```python
from build123d import *

# Parameters (mm, degrees)
SKETCH2_W                                           = 70
SKETCH2_H                                           = 115
BOSS_EXTRUDE1_DEPTH                                 = 10
SKETCH8_W                                           = 70
SKETCH8_H                                           = 77
SKETCH8_W_2                                         = 44
SKETCH8_H_2                                         = 59
BOSS_EXTRUDE5_DEPTH                                 = 50
SKETCH9_R                                           = 4
CUT_EXTRUDE1_DEPTH                                  = 50
CUT_EXTRUDE2_REACH                                  = 107.948
SKETCH10_W                                          = 25
SKETCH10_H                                          = 25
CSK_FOR_M3_COUNTERSUNK_FLAT_HEAD_SCREW1_D           = 3.4
CSK_FOR_M3_COUNTERSUNK_FLAT_HEAD_SCREW1_DEPTH       = 5
CSK_FOR_M3_COUNTERSUNK_FLAT_HEAD_SCREW1_CSINK_D     = 6.3
CSK_FOR_M3_COUNTERSUNK_FLAT_HEAD_SCREW1_CSINK_ANGLE = 90
FILLET1_R                                           = 2
CSK_FOR_M3_COUNTERSUNK_FLAT_HEAD_SCR_2_COUNT        = 2
CSK_FOR_M3_COUNTERSUNK_FLAT_HEAD_SCR_2_PITCH        = 59.993922781
CSK_FOR_M3_COUNTERSUNK_FLAT_HEAD_SCR_3_COUNT        = 2
CSK_FOR_M3_COUNTERSUNK_FLAT_HEAD_SCR_3_PITCH        = 84.983361201
CSK_FOR_M3_COUNTERSUNK_FLAT_HEAD_SCR_4_COUNT        = 2
CSK_FOR_M3_COUNTERSUNK_FLAT_HEAD_SCR_4_PITCH        = 102.955177918
CSK_FOR_M3_COUNTERSUNK_FLAT_HEAD_SCR_5_COUNT        = 2
CSK_FOR_M3_COUNTERSUNK_FLAT_HEAD_SCR_5_PITCH        = 118.101251225
CSK_FOR_M3_COUNTERSUNK_FLAT_HEAD_SCR_6_COUNT        = 2
CSK_FOR_M3_COUNTERSUNK_FLAT_HEAD_SCR_6_PITCH        = 102.856688561
CSK_FOR_M5_COUNTERSUNK_FLAT_HEAD_SCREW2_D           = 5.5
CSK_FOR_M5_COUNTERSUNK_FLAT_HEAD_SCREW2_DEPTH       = 30
CSK_FOR_M5_COUNTERSUNK_FLAT_HEAD_SCREW2_CSINK_D     = 10.4
CSK_FOR_M5_COUNTERSUNK_FLAT_HEAD_SCREW2_CSINK_ANGLE = 90
CSK_FOR_M5_COUNTERSUNK_FLAT_HEAD_SCREW2_TIP         = 1.652366702


with BuildPart() as part:
    # Sketch2 → Boss-Extrude1 (new body)
    with BuildSketch(Plane(origin=(0, 0, 0), x_dir=(1, 0, 0), z_dir=(0, 1, 0))):
        with Locations((0, 7.5)):
            Rectangle(SKETCH2_W, SKETCH2_H)
    extrude(amount=BOSS_EXTRUDE1_DEPTH)

    # Sketch8 → Boss-Extrude5 (add)
    with BuildSketch(Plane(origin=(0, 10, 0), x_dir=(1, 0, 0), z_dir=(0, 1, 0))):
        with Locations((0, 18.5)):
            Rectangle(SKETCH8_W, SKETCH8_H)
        with Locations((0, 14.5)):
            Rectangle(SKETCH8_W_2, SKETCH8_H_2, mode=Mode.SUBTRACT)
    extrude(amount=BOSS_EXTRUDE5_DEPTH)

    # Sketch9 → Cut-Extrude1 (cut)
    with BuildSketch(Plane(origin=(0, 60, 0), x_dir=(1, 0, 0), z_dir=(0, 1, 0))):
        with Locations(Location((-28.5, 50.5, 0), (0, 0, 270))):
            Circle(SKETCH9_R)
        with Locations(Location((28.5, 50.5, 0), (0, 0, 270))):
            Circle(SKETCH9_R)
        with Locations(Location((28.5, -13.5, 0), (0, 0, 270))):
            Circle(SKETCH9_R)
        with Locations(Location((-28.5, -13.5, 0), (0, 0, 270))):
            Circle(SKETCH9_R)
    extrude(amount=-CUT_EXTRUDE1_DEPTH, mode=Mode.SUBTRACT)

    # Sketch10 → Cut-Extrude2 (cut, up to next)
    with BuildSketch(Plane(origin=(0, 0, 15), x_dir=(-1, 0, 0), z_dir=(0, 0, -1)), mode=Mode.PRIVATE) as cut_extrude2_sk1:
        with Locations((0, 32)):
            Rectangle(SKETCH10_W, SKETCH10_H)
    cut_extrude2_tool1 = extrude(cut_extrude2_sk1.sketch, amount=-CUT_EXTRUDE2_REACH, mode=Mode.PRIVATE) & part.part
    add(cut_extrude2_tool1.solids().sort_by_distance((0, 32, 15))[0], mode=Mode.SUBTRACT)

    # CSK for M3 Countersunk Flat Head Screw1
    with Locations(Plane.XY.offset(20)):
        with Locations((-15.5, 47.5), (15.5, 47.5), (15.5, 16.5), (-15.5, 16.5)):
            CounterSinkHole(CSK_FOR_M3_COUNTERSUNK_FLAT_HEAD_SCREW1_D / 2, CSK_FOR_M3_COUNTERSUNK_FLAT_HEAD_SCREW1_CSINK_D / 2, depth=CSK_FOR_M3_COUNTERSUNK_FLAT_HEAD_SCREW1_DEPTH, counter_sink_angle=CSK_FOR_M3_COUNTERSUNK_FLAT_HEAD_SCREW1_CSINK_ANGLE)

    # Fillet1
    fillet1_edges = [part.edges().sort_by_distance(p)[0] for p in [
        (-35, 10, -61),
        (35, 10, -61),
        (-35, 10, 35),
        (0, 10, 50),
        (-35, 35, 20),
        (35, 35, 20),
        (0, 60, -57),
        (35, 35, -57),
        (-35, 35, -57),
        (0, 60, 20),
        (35, 60, -18.5),
        (-35, 60, -18.5),
        (35, 10, 35),
        (35, 5, 50),
        (-35, 5, 50),
        (-35, 5, -65),
        (35, 5, -65),
        (0, 10, -65),
    ]]
    fillet(fillet1_edges, radius=FILLET1_R)

    # Sketch18 → CSK for M3 Countersunk Flat Head Screw2 (revolve, cut)
    with BuildSketch(Plane(origin=(-29.898999739, 10, -59.914683203), x_dir=(0, 0, 1), z_dir=(1, 0, 0))):
        Polygon((0, 0), (0, 31.021463052), (1.7, 30), (1.7, 1.45), (3.15, 0), align=None)
    csk_for_m3_countersunk_flat_head_screw2 = revolve(axis=Axis((-29.898999739, 16.35, -59.914683203), (0, -1, 0)), mode=Mode.SUBTRACT)

    # CSK for M3 Countersunk Flat Head Scr 2: CSK for M3 Countersunk Flat Head Screw2 ×2
    with Locations(*[Vector(0.999999912683058, 0, 0.00041789218284246394) * (i * CSK_FOR_M3_COUNTERSUNK_FLAT_HEAD_SCR_2_PITCH) for i in range(1, CSK_FOR_M3_COUNTERSUNK_FLAT_HEAD_SCR_2_COUNT)]):
        add(csk_for_m3_countersunk_flat_head_screw2, mode=Mode.SUBTRACT)

    # CSK for M3 Countersunk Flat Head Scr 3: CSK for M3 Countersunk Flat Head Screw2 ×2
    with Locations(*[Vector(0.023234335515626516, 0, 0.9997300463890977) * (i * CSK_FOR_M3_COUNTERSUNK_FLAT_HEAD_SCR_3_PITCH) for i in range(1, CSK_FOR_M3_COUNTERSUNK_FLAT_HEAD_SCR_3_COUNT)]):
        add(csk_for_m3_countersunk_flat_head_screw2, mode=Mode.SUBTRACT)

    # CSK for M3 Countersunk Flat Head Scr 4: CSK for M3 Countersunk Flat Head Screw2 ×2
    with Locations(*[Vector(0.5634477960813598, 0, 0.8261516695444358) * (i * CSK_FOR_M3_COUNTERSUNK_FLAT_HEAD_SCR_4_PITCH) for i in range(1, CSK_FOR_M3_COUNTERSUNK_FLAT_HEAD_SCR_4_COUNT)]):
        add(csk_for_m3_countersunk_flat_head_screw2, mode=Mode.SUBTRACT)

    # CSK for M3 Countersunk Flat Head Scr 5: CSK for M3 Countersunk Flat Head Screw2 ×2
    with Locations(*[Vector(0.4905385745621895, 0, 0.8714194781312243) * (i * CSK_FOR_M3_COUNTERSUNK_FLAT_HEAD_SCR_5_PITCH) for i in range(1, CSK_FOR_M3_COUNTERSUNK_FLAT_HEAD_SCR_5_COUNT)]):
        add(csk_for_m3_countersunk_flat_head_screw2, mode=Mode.SUBTRACT)

    # CSK for M3 Countersunk Flat Head Scr 6: CSK for M3 Countersunk Flat Head Screw2 ×2
    with Locations(*[Vector(0.01850192219633628, 0, 0.9998288247870436) * (i * CSK_FOR_M3_COUNTERSUNK_FLAT_HEAD_SCR_6_PITCH) for i in range(1, CSK_FOR_M3_COUNTERSUNK_FLAT_HEAD_SCR_6_COUNT)]):
        add(csk_for_m3_countersunk_flat_head_screw2, mode=Mode.SUBTRACT)

    # CSK for M5 Countersunk Flat Head Screw2
    with Locations(Plane(origin=(0, 10, 0), x_dir=(1, 0, 0), z_dir=(0, 1, 0))):
        with Locations((0.174986864, 14.411981132)):
            CounterSinkHole(CSK_FOR_M5_COUNTERSUNK_FLAT_HEAD_SCREW2_D / 2, CSK_FOR_M5_COUNTERSUNK_FLAT_HEAD_SCREW2_CSINK_D / 2, depth=CSK_FOR_M5_COUNTERSUNK_FLAT_HEAD_SCREW2_DEPTH, counter_sink_angle=CSK_FOR_M5_COUNTERSUNK_FLAT_HEAD_SCREW2_CSINK_ANGLE)
            with Locations((0, 0, -(CSK_FOR_M5_COUNTERSUNK_FLAT_HEAD_SCREW2_DEPTH + CSK_FOR_M5_COUNTERSUNK_FLAT_HEAD_SCREW2_TIP / 2))):  # 118° drill point
                Cone(0, CSK_FOR_M5_COUNTERSUNK_FLAT_HEAD_SCREW2_D / 2, CSK_FOR_M5_COUNTERSUNK_FLAT_HEAD_SCREW2_TIP, mode=Mode.SUBTRACT)


solid = part.part
```
Work out the finished part from the listing and answer in its coordinate system (mm). A direction names the side the tool comes from. Coordinates: 2 decimals unless noted, no trailing zeros. Order: outer loops, then holes, each group sorted by start corner. A loop starts at its lowest first (then second) coordinate and runs counter-clockwise, first axis right, second up. Notation, with made-up numbers: (46.25, -37.75) - (64.25, -37.75) arc R6 ccw to (64.25, -32.75) - close; hole circle Ø8 at (33, 18). An arc over 180 degrees is marked (long way). Answer as a JSON object with one key per item and string values.
1. Find section A-A on y = 47.5. Determine the outline of the cut face in (x, z), plus the area to 3 significant figures.
Output values:
{"outline": "(-35, -55) arc R2 ccw to (-33, -57) - (33, -57) arc R2 ccw to (35, -55) - (35, 18) arc R2 ccw to (33, 20) - (18.65, 20) - (17.2, 18.55) - (17.2, 15) - (22, 15) - (22, -44) - (-22, -44) - (-22, 15) - (-17.2, 15) - (-17.2, 18.55) - (-18.65, 20) - (-33, 20) arc R2 ccw to (-35, 18) - close; (-13.8, 15) - (13.8, 15) - (13.8, 18.55) - (12.35, 20) - (-12.35, 20) - (-13.8, 18.55) - close; hole circle Ø8 at (-28.5, -50.5); hole circle Ø8 at (-28.5, 13.5); hole circle Ø8 at (28.5, -50.5); hole circle Ø8 at (28.5, 13.5)", "area": "2,550 mm²"}
2. The mould has two halves that part along X. Classify faces 1 (the face through (-25.8, 35.35, 10.55)), 2 (the face through (0, 4, -65)), 3 (the face through (0, 44.5, 17)): +X half, -X half, draft (parallel to the pull), parting line (faces both ways), or undercut.
Output values:
{"face 1": "undercut", "face 2": "draft", "face 3": "undercut"}
3. Consider line 1 (Y direction, x = 15.5, z = 16.1); line 2 (X direction, y = 55.5, z = -14); line 3 (Z direction, x = -32, y = 46). Determine where each line is inside the solid, lowest interval first.
Output values:
{"line 1": "y = 0 to 14.8, 18.2 to 45.8, 49.2 to 60", "line 2": "x = -35 to -22, 22 to 35", "line 3": "z = -57 to -52.44, -48.56 to 11.56, 15.44 to 20"}
4. Find section D-D on x = 16. Count the separate pieces of the cut face and the enclosed holes in it, plus the area to 3 significant figures.
Output values:
{"separate pieces": "3", "enclosed holes": "0", "area": "2,010 mm²"}
5. A tool of negligible diameter and unlimited length cuts with its end or side. For faces 4 (the face through (29.619, 4.335, 25.926)), 5 (the face through (29, 10, 13)), 6 (the face through (0, 19.5, 17)), from which of +Z, -Z, +X, -X, +Y, -Y can it reach the whole face along a straight path? Write none if from no direction.
Output values:
{"face 4": "+Y, -Y", "face 5": "+Y", "face 6": "+Z"}
6. Each of these flat-tipped pins is pushed along its axis until it touches: P1, Ø3, axis at x = 17, y = 36.5, coming from the -Z side; P2, Ø2, axis at x = -5, z = -20.5, coming from the +Y side; P3, Ø5, axis at x = 23.5, y = 11, coming from the -Z side. Where does it stop, or does it pass through?
Output values:
{"P1": "stops at z = -57", "P2": "stops at y = 10", "P3": "stops at z = -64.94"}
7. Find section B-B on x = -15.5. Determine the outline of the cut face in (y, z).
Output values:
{"outline": "(0, -65) - (8, -65) arc R2 ccw to (10, -63) - (10, -57) - (58, -57) arc R2 ccw to (60, -55) - (60, -44) - (10, -44) - (10, 15) - (14.8, 15) - (14.8, 18.55) - (13.35, 20) - (10, 20) - (10, 48) arc R2 ccw to (8, 50) - (0, 50) - close; (18.2, 15) - (45.8, 15) - (45.8, 18.55) - (44.35, 20) - (19.65, 20) - (18.2, 18.55) - close; (49.2, 15) - (60, 15) - (60, 18) arc R2 ccw to (58, 20) - (50.65, 20) - (49.2, 18.55) - close"}
8. Find section C-C on z = -40.5. Determine the outline of the cut face in (x, y).
Output values:
{"outline": "(-35, 0) - (35, 0) - (35, 58) arc R2 ccw to (33, 60) - (22, 60) - (22, 10) - (-22, 10) - (-22, 60) - (-33, 60) arc R2 ccw to (-35, 58) - close"}
